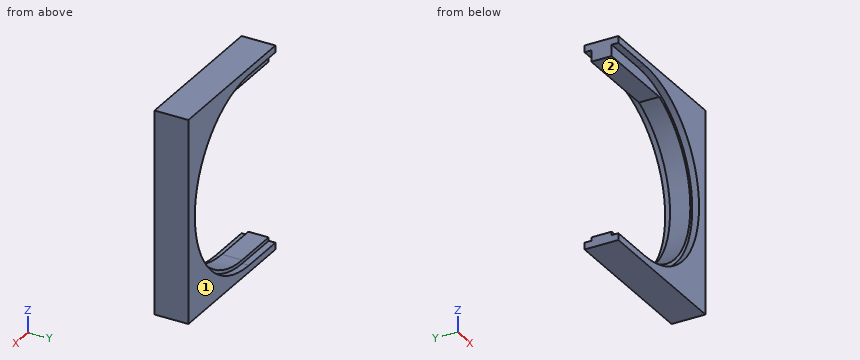
from build123d import *

# Parameters (mm, degrees)
BOSS_EXTRUDE1_DEPTH = 3.81
BOSS_EXTRUDE2_DEPTH = 2.286


with BuildPart() as part:
    # Sketch1 → Boss-Extrude1 (new, symmetric)
    with BuildSketch(Plane(origin=(0, 0, 0), x_dir=(1, 0, 0), z_dir=(0, 1, 0))):
        with BuildLine():
            Line((0, 45.72), (0, 44.196))
            Line((0, 44.196), (10.414, 44.196))
            ThreePointArc((10.414, 44.196), (31.75, 22.86), (10.414, 1.524))
            Line((10.414, 1.524), (0, 1.524))
            Line((0, 1.524), (0, 0))
            Line((0, 0), (34.29, 0))
            Line((34.29, 0), (34.29, 45.72))
            Line((34.29, 45.72), (0, 45.72))
        make_face()
    extrude(amount=BOSS_EXTRUDE1_DEPTH, both=True)

    # Sketch2 → Boss-Extrude2 (add, symmetric)
    with BuildSketch(Plane(origin=(0, 0, 0), x_dir=(1, 0, 0), z_dir=(0, 1, 0))):
        with BuildLine():
            Line((0, 4.064), (18.780591899, 4.064))
            ThreePointArc((18.780591899, 4.064), (30.538591673, 27.136714393), (10.414, 43.434))
            Line((10.414, 43.434), (0, 43.434))
            Line((0, 43.434), (0, 44.196))
            Line((0, 44.196), (10.414, 44.196))
            ThreePointArc((10.414, 44.196), (31.75, 22.86), (10.414, 1.524))
            Line((10.414, 1.524), (0, 1.524))
            Line((0, 1.524), (0, 4.064))
        make_face()
    extrude(amount=BOSS_EXTRUDE2_DEPTH, both=True)


solid = part.part
The listing builds one solid part. Answer for the finished solid, in the listing's coordinates (mm). Face numbers are marked on the shaded views. A direction names the side the tool comes from. Round coordinates to 2 decimals unless told otherwise and drop trailing zeros. Write each loop counter-clockwise with the first axis right and the second up, starting at its lowest first coordinate (ties: lowest second). Pieces come first, ordered by that corner, then holes. Notation, with made-up numbers: M -13,-25.75 L 24,-25.75 A32 cw 24,10.25 Z; hole C 11.25,-14.5 d10. An arc over 180 degrees is marked long. Write each question's results on one line, items separated by ' | '. Start each with the question number.
Item 1: Flat-ended cylindrical pins translate along their axes: pin 1 Ø10 at (x, z) = (20, -17) entering from -Y; pin 2 Ø0.5 at (x, y) = (7, -3) entering from +Z. Find the tip coordinate at first contact, or state that the pin passes through.
Item 2: A cutting plane is placed at A-A on x = 8. Write down the section's boundary in (y, z), and give its area (3 significant figures).
Item 3: A cutting plane is placed at B-B on y = 3. Write down the section's boundary in (x, z), and give its area (3 significant figures).
Item 4: For the marked faces 1 and 2, determine the directions among +Z, -Z, +X, -X, +Y, -Y from which every point of the face is accessible in a straight line to the end or side of a thin tool.
Item 5: A cutting plane is placed at D-D on x = 16. Write down the section's boundary in (y, z), and give its area (3 significant figures).
Item 6: Straight lines are drawn through the part: L1, parallel to Z at x = 3.5, y = 3.75; L2, parallel to Z at x = 3, y = 0; L3, parallel to X at y = 2.25, z = -39. For each, find the intervals that lie inside material, in ascending order. Write a range as [from, to].
Item 7: A cutting plane is placed at C-C on z = -22.86. Write down the section's boundary in (x, y), and give its area (3 significant figures).
Check sheet entries:
1) pin 1: through | pin 2: z = 0
2) outline: M -3.81,-45.72 L 3.81,-45.72 L 3.81,-44.2 L 2.29,-44.2 L 2.29,-43.43 L -2.29,-43.43 L -2.29,-44.2 L -3.81,-44.2 Z; M -3.81,-1.52 L -2.29,-1.52 L -2.29,-4.06 L 2.29,-4.06 L 2.29,-1.52 L 3.81,-1.52 L 3.81,0 L -3.81,0 Z | area: 38.3 mm²
3) outline: M 0,-45.72 L 34.29,-45.72 L 34.29,0 L 0,0 L 0,-1.52 L 10.41,-1.52 A21.34 cw 10.41,-44.2 L 0,-44.2 Z | area: 408 mm²
4) face 1: +Z, -Z, +X, -X, +Y | face 2: -X, +Y, -Y
5) outline: M -3.81,-45.72 L 3.81,-45.72 L 3.81,-43.45 L 2.29,-43.45 L 2.29,-42.66 L -2.29,-42.66 L -2.29,-43.45 L -3.81,-43.45 Z; M -3.81,-2.27 L -2.29,-2.27 L -2.29,-4.06 L 2.29,-4.06 L 2.29,-2.27 L 3.81,-2.27 L 3.81,0 L -3.81,0 Z | area: 46.4 mm²
6) L1: [-45.72, -44.2], [-1.52, 0] | L2: [-45.72, -43.43], [-4.06, 0] | L3: [23.17, 34.29]
7) outline: M 30.99,-2.29 L 31.75,-2.29 L 31.75,-3.81 L 34.29,-3.81 L 34.29,3.81 L 31.75,3.81 L 31.75,2.29 L 30.99,2.29 Z | area: 22.8 mm²
